Can you work these out from the model? Positions are in its coordinate system, mm. A direction names the side the tool comes from. Give positions to 0.01 mm unless a question says otherwise; leave off trailing zeros. Order: outer loops, then holes, each group sorted by start corner. A loop starts at its lowest first (then second) coordinate and runs counter-clockwise, first axis right, second up. Notation, with made-up numbers: (51.25, -39) - (102.25, -39) arc R37 ccw to (102.25, -1) - close; hole circle Ø4 at (-29, -18.75). An arc over 180 degrees is marked (long way). Use one line per item in the form item = value. Start each with the question number.
1) Suppose I cut it at C-C, the plane y = 17.5. Write out the boundary of the cut face in (x, z) (3 decimals), and give its area (3 significant figures).
2) Suppose I cut it at B-B, the plane y = 29.5. Write out the boundary of the cut face in (x, z), and give its area (3 significant figures).
3) Suppose I cut it at A-A, the plane x = 0. Write out the boundary of the cut face in (y, z).
4) For pin 1 (1.1 mm diameter, centred on x = 89, y = 10, fed in from -Z) (3 decimals); pin 2 (10 mm diameter, centred on y = 17.5, z = -53.5, fed in from -X); pin 3 (1.5 mm diameter, centred on y = 2.5, z = -26.5, fed in from -X), each with a flat end and sliding along its axis, tell me the tip position at first contact or that it passes through.
5) Suppose I cut it at D-D, the plane x = -66. Write out the boundary of the cut face in (y, z).
6) We'd pull the mould along X, two halves only. Please class faces 1 (the flat face through (40.97, 44.89, 38.82)), 2 (the cylindrical face through (26.135, 38.173, 30.251)), 3 (the flat face through (13, 24, -15)): released by +X, released by -X, zero draft, split by the parting line, or undercut.
7) Please list where these lines run through material, in increasing order: probe 1 along Y at (x, z) = (-88.15, 0); probe 2 along Z at (x, y) = (0, 1); probe 3 along Z at (x, y) = (11, 38.5).
8) Which directions (+Z, -Z, +X, -X, +Y, -Y) give clear straight access to the entire face, cutting with the end or side of a thin tool? Please do faces 4 (the flat face through (-13.06, 2.5, 7.38)), 5 (the flat face through (-31.11, 17.15, -0.92)), 6 (the flat face through (-87.122, 7, 0)), 7 (the flat face through (13.13, 44.97, -17.58)).
```python
from build123d import *

# Parameters (mm, degrees)
SKETCH1_R           = 10
BASE_DEPTH          = 5.08
SKETCH2_R           = 12
SKETCH2_R_2         = 1.5
MOTOREXTRUDE_DEPTH  = 6.35
CIRPATTERN3_COUNT   = 3
CIRPATTERN3_ANGLE   = 240
BOSS_EXTRUDE1_DEPTH = 12.7
SKETCH3_R           = 1.5
CUT_EXTRUDE1_DEPTH  = 5.018


with BuildPart() as part:
    # Sketch1 → Base (new body)
    with BuildSketch(Plane(origin=(0, 0, 0), x_dir=(1, 0, 0), z_dir=(0, 1, 0))):
        with BuildLine():
            Line((-10, 15), (-10, 57.3926))
            Line((-10, 57.3926), (-15, 57.3926))
            Line((-15, 57.3926), (-15, 89.897161246))
            ThreePointArc((-15, 89.897161246), (-78.929555301, 45.57), (-85.353225367, -31.958199566))
            Line((-85.353225367, -31.958199566), (-57.203449589, -15.705918943))
            Line((-57.203449589, -15.705918943), (-54.703449589, -20.036045962))
            Line((-54.703449589, -20.036045962), (-17.990381057, 1.160254038))
            Line((-17.990381057, 1.160254038), (-7.990381057, -16.160254038))
            Line((-7.990381057, -16.160254038), (-44.703449589, -37.356554038))
            Line((-44.703449589, -37.356554038), (-42.203449589, -41.686681057))
            Line((-42.203449589, -41.686681057), (-70.353225367, -57.93896168))
            ThreePointArc((-70.353225367, -57.93896168), (0, -91.14), (70.353225367, -57.93896168))
            Line((70.353225367, -57.93896168), (42.203449589, -41.686681057))
            Line((42.203449589, -41.686681057), (44.703449589, -37.356554038))
            Line((44.703449589, -37.356554038), (7.990381057, -16.160254038))
            Line((7.990381057, -16.160254038), (17.990381057, 1.160254038))
            Line((17.990381057, 1.160254038), (54.703449589, -20.036045962))
            Line((54.703449589, -20.036045962), (57.203449589, -15.705918943))
            Line((57.203449589, -15.705918943), (85.353225367, -31.958199566))
            ThreePointArc((85.353225367, -31.958199566), (78.929555301, 45.57), (15, 89.897161246))
            Line((15, 89.897161246), (15, 57.3926))
            Line((15, 57.3926), (10, 57.3926))
            Line((10, 57.3926), (10, 15))
            Line((10, 15), (-10, 15))
        make_face()
        Circle(SKETCH1_R, mode=Mode.SUBTRACT)
    extrude(amount=BASE_DEPTH)

    # Sketch2 → MotorExtrude (add)
    with BuildSketch(Plane(origin=(-5, 0, 8.660254038), x_dir=(-0.866025404, 0, -0.5), z_dir=(0.5, 0, -0.866025404))):
        Polygon((-15, 5.08), (-57.3926, 5.08), (-57.3926, 42.39), (-52.3126, 47.47), (-20.08, 47.47), (-15, 42.39), align=None)
        with Locations((-36.1963, 26.275)):
            Circle(SKETCH2_R, mode=Mode.SUBTRACT)
        with Locations((-20.701824858, 41.768524843)):
            Circle(SKETCH2_R_2, mode=Mode.SUBTRACT)
        with Locations((-20.702775157, 10.780524858)):
            Circle(SKETCH2_R_2, mode=Mode.SUBTRACT)
        with Locations((-51.690775142, 10.781475157)):
            Circle(SKETCH2_R_2, mode=Mode.SUBTRACT)
        with Locations((-51.689824843, 41.769475142)):
            Circle(SKETCH2_R_2, mode=Mode.SUBTRACT)
    motorextrude = extrude(amount=-MOTOREXTRUDE_DEPTH)

    # CirPattern3: MotorExtrude ×3 about axis
    cirpattern3_axis = Axis((0, 0, 0), (0, 1, 0))
    for i in range(1, CIRPATTERN3_COUNT):
        add(motorextrude.rotate(cirpattern3_axis, i * CIRPATTERN3_ANGLE / (CIRPATTERN3_COUNT - 1)))

    # Sketch1<7> → Boss-Extrude1 (add)
    with BuildSketch(Plane(origin=(0, 0, 0), x_dir=(1, 0, 0), z_dir=(0, 1, 0))):
        with BuildLine():
            Line((-87.122, 9.525), (-90.640906742, 9.525))
            ThreePointArc((-90.640906742, 9.525), (-91.14, 0), (-90.640906742, -9.525))
            Line((-90.640906742, -9.525), (-87.122, -9.525))
            Line((-87.122, -9.525), (-87.122, 9.525))
        make_face()
        with BuildLine():
            Line((87.122, 9.525), (87.122, -9.525))
            Line((87.122, -9.525), (90.640906742, -9.525))
            ThreePointArc((90.640906742, -9.525), (91.14, 0), (90.640906742, 9.525))
            Line((90.640906742, 9.525), (87.122, 9.525))
        make_face()
    extrude(amount=BOSS_EXTRUDE1_DEPTH)

    # Sketch3 → Cut-Extrude1 (cut, through all)
    with BuildSketch(Plane.ZY.offset(-87.122)):
        with Locations((0, 8.89)):
            Circle(SKETCH3_R)
    cut_extrude1 = extrude(amount=-CUT_EXTRUDE1_DEPTH, mode=Mode.SUBTRACT)

    # Mirror1: Cut-Extrude1 across plane
    add(cut_extrude1.mirror(Plane(origin=(0, 0, 0), x_dir=(0, 0, 1), z_dir=(1, 0, 0))), mode=Mode.SUBTRACT)


solid = part.part
```
Result sheet:
q1.outline = (-57.878, 14.537) - (-46.611, 8.031) - (-43.436, 13.531) - (-54.703, 20.036) - close; (-32.433, -0.154) - (-21.165, -6.66) - (-17.99, -1.16) - (-29.258, 5.345) - close; (4.815, 21.66) - (7.99, 16.16) - (19.258, 22.666) - (16.083, 28.165) - close; (10, -57.393) - (16.35, -57.393) - (16.35, -44.382) - (10, -44.382) - close; (10, -28.011) - (16.35, -28.011) - (16.35, -15) - (10, -15) - close; (30.261, 36.35) - (33.436, 30.851) - (44.703, 37.357) - (41.528, 42.856) - close
q1.area = 496 mm²
q2.outline = (-57.88, 14.54) - (-49.53, 9.72) - (-46.36, 15.22) - (-54.7, 20.04) - close; (-29.51, -1.84) - (-21.17, -6.66) - (-17.99, -1.16) - (-26.34, 3.66) - close; (4.82, 21.66) - (7.99, 16.16) - (16.34, 20.98) - (13.16, 26.48) - close; (10, -57.39) - (16.35, -57.39) - (16.35, -47.75) - (10, -47.75) - close; (10, -24.64) - (16.35, -24.64) - (16.35, -15) - (10, -15) - close; (33.18, 38.04) - (36.36, 32.54) - (44.7, 37.36) - (41.53, 42.86) - close
q2.area = 367 mm²
q3.outline = (0, -15) - (5.08, -15) - (5.08, -10) - (0, -10) - close; (0, 10) - (5.08, 10) - (5.08, 91.14) - (0, 91.14) - close
q4.pin_1 = -9.525
q4.pin_2 = 10
q4.pin_3 = -87.43
q5.outline = (0, -62.85) - (5.08, -62.85) - (5.08, 20.78) - (0, 20.78) - close; (0, 55.43) - (5.08, 55.43) - (5.08, 62.85) - (0, 62.85) - close
q6.face_1 = released by +X
q6.face_2 = undercut
q6.face_3 = zero draft
q7.probe_1 = 0 to 7.39, 10.39 to 12.7
q7.probe_2 = -15 to -10, 10 to 91.14
q7.probe_3 = -57.39 to -15, 17.9 to 25.23
q8.face_4 = +Y, -Y
q8.face_5 = -Z, +Y
q8.face_6 = +Z, -Z, +Y
q8.face_7 = +X, -X, +Y
